Work out the finished part from the listing and answer in its coordinate system (mm). A direction names the side the tool comes from. Round coordinates to 2 decimals unless told otherwise and drop trailing zeros. Loops run counter-clockwise (first coordinate to the right, second up) from the corner with the lowest first, then second, coordinate; pieces in that order, holes last. Notation, with made-up numbers: (17, 3) - (44, 3) arc R30 cw to (44, 25) - close; hole circle Ø7 at (-27, 57.5). An arc over 180 degrees is marked (long way). Return JSON: item names as keys, results as strings.
from build123d import *

# Parameters (mm, degrees)
SKETCH1_W             = 50
SKETCH1_H             = 50
BOSS_EXTRUDE1_DEPTH   = 1810
BOSS_EXTRUDE1_2_DEPTH = 1810
BOSS_EXTRUDE1_3_DEPTH = 1810
BOSS_EXTRUDE1_4_DEPTH = 1810
BOSS_EXTRUDE2_START   = 10
SKETCH2_W             = 50
SKETCH2_H             = 750
SKETCH2_W_2           = 750
SKETCH2_H_2           = 100
BOSS_EXTRUDE2_DEPTH   = 180
SKETCH4_W             = 750
SKETCH4_H             = 110
CUT_EXTRUDE4_DEPTH    = 1050
SKETCH5_W             = 50
SKETCH5_H             = 50
SKETCH5_H_2           = 60
BOSS_EXTRUDE3_DEPTH   = 770
SKETCH6_W             = 50
SKETCH6_H             = 60
BOSS_EXTRUDE4_DEPTH   = 770
SKETCH8_W             = 50
SKETCH8_H             = 50
BOSS_EXTRUDE5_DEPTH   = 770
SKETCH9_W             = 50
SKETCH9_H             = 30
BOSS_EXTRUDE6_DEPTH   = 770
SKETCH10_R            = 15
BOSS_EXTRUDE7_DEPTH   = 770
SKETCH11_W            = 50
SKETCH11_H            = 30
BOSS_EXTRUDE8_DEPTH   = 770
SKETCH12_W            = 50
SKETCH12_H            = 30
BOSS_EXTRUDE9_DEPTH   = 770


with BuildPart() as part:
    # Sketch1 → Boss-Extrude1 (new body)
    with BuildSketch(Plane(origin=(0, 0, 0), x_dir=(1, 0, 0), z_dir=(0, 1, 0))):
        with Locations((-427.760736196, -623.312883436)):
            Rectangle(SKETCH1_W, SKETCH1_H)
    extrude(amount=BOSS_EXTRUDE1_DEPTH)



with BuildPart() as body_2:
    # Sketch1 → Boss-Extrude1 2 (new body)
    with BuildSketch(Plane(origin=(0, 0, 0), x_dir=(1, 0, 0), z_dir=(0, 1, 0))):
        with Locations((372.239263804, -623.312883436)):
            Rectangle(SKETCH1_W, SKETCH1_H)
    extrude(amount=BOSS_EXTRUDE1_2_DEPTH)


with BuildPart() as body_3:
    # Sketch1 → Boss-Extrude1 3 (new body)
    with BuildSketch(Plane(origin=(0, 0, 0), x_dir=(1, 0, 0), z_dir=(0, 1, 0))):
        with Locations((372.239263804, 176.687116564)):
            Rectangle(SKETCH1_W, SKETCH1_H)
    extrude(amount=BOSS_EXTRUDE1_3_DEPTH)


with BuildPart() as body_4:
    # Sketch1 → Boss-Extrude1 4 (new body)
    with BuildSketch(Plane(origin=(0, 0, 0), x_dir=(1, 0, 0), z_dir=(0, 1, 0))):
        with Locations((-427.760736196, 176.687116564)):
            Rectangle(SKETCH1_W, SKETCH1_H)
    extrude(amount=BOSS_EXTRUDE1_4_DEPTH)


with BuildPart() as part_1:
    add(part.part)

    add(body_2.part)  # Boss-Extrude2 merges body 2

    add(body_3.part)  # Boss-Extrude2 merges body 3

    add(body_4.part)  # Boss-Extrude2 merges body 4
    # Sketch2 → Boss-Extrude2 (add)
    with BuildSketch(Plane(origin=(0, 0, 0), x_dir=(-1, 0, 0), z_dir=(0, -1, 0)).offset(BOSS_EXTRUDE2_START)):
        with Locations((427.760736196, -223.312883436)):
            Rectangle(SKETCH2_W, SKETCH2_H)
        with Locations((27.760736196, -223.312883436)):
            Rectangle(SKETCH2_W_2, SKETCH2_H_2)
        with Locations((-372.239263804, -223.312883436)):
            Rectangle(SKETCH2_W, SKETCH2_H)
    extrude(amount=-BOSS_EXTRUDE2_DEPTH)

    # Sketch4 → Cut-Extrude4 (cut)
    with BuildSketch(Plane.ZY.offset(452.760736196)):
        with Locations((223.312883436, 45)):
            Rectangle(SKETCH4_W, SKETCH4_H)
    extrude(amount=-CUT_EXTRUDE4_DEPTH, mode=Mode.SUBTRACT)

    # Sketch5 → Boss-Extrude3 (add)
    with BuildSketch(Plane.ZY.offset(-347.239263804)):
        with Locations((-176.687116564, 940)):
            Rectangle(SKETCH5_W, SKETCH5_H)
        with Locations((623.312883436, 935)):
            Rectangle(SKETCH5_W, SKETCH5_H_2)
    extrude(amount=BOSS_EXTRUDE3_DEPTH)

    # Sketch6 → Boss-Extrude4 (add)
    with BuildSketch(Plane(origin=(0, 0, 598.312883436), x_dir=(-1, 0, 0), z_dir=(0, 0, -1))):
        with Locations((-372.239263804, 935)):
            Rectangle(SKETCH6_W, SKETCH6_H)
        with Locations((427.760736196, 935)):
            Rectangle(SKETCH6_W, SKETCH6_H)
    extrude(amount=BOSS_EXTRUDE4_DEPTH)

    # Sketch8 → Boss-Extrude5 (add)
    with BuildSketch(Plane(origin=(0, 0, 598.312883436), x_dir=(-1, 0, 0), z_dir=(0, 0, -1))):
        with Locations((-372.239263804, 1514.740067664)):
            Rectangle(SKETCH8_W, SKETCH8_H)
        with Locations((427.760736196, 1514.740067664)):
            Rectangle(SKETCH8_W, SKETCH8_H)
    extrude(amount=BOSS_EXTRUDE5_DEPTH)

    # Sketch9 → Boss-Extrude6 (add)
    with BuildSketch(Plane.XY.offset(-151.687116564)):
        with Locations((-427.760736196, 1795)):
            Rectangle(SKETCH9_W, SKETCH9_H)
        with Locations((372.239263804, 1795)):
            Rectangle(SKETCH9_W, SKETCH9_H)
    extrude(amount=BOSS_EXTRUDE6_DEPTH)

    # Sketch10 → Boss-Extrude7 (add)
    with BuildSketch(Plane(origin=(-402.760736196, 0, 0), x_dir=(0, 0, -1), z_dir=(1, 0, 0))):
        with Locations(Location((-223.312883436, 1795, 0), (0, 0, 270))):
            Circle(SKETCH10_R)
    extrude(amount=BOSS_EXTRUDE7_DEPTH)

    # Sketch11 → Boss-Extrude8 (add)
    with BuildSketch(Plane.ZY.offset(-347.239263804)):
        with Locations((-176.687116564, 1795)):
            Rectangle(SKETCH11_W, SKETCH11_H)
    extrude(amount=BOSS_EXTRUDE8_DEPTH)

    # Sketch12 → Boss-Extrude9 (add)
    with BuildSketch(Plane.ZY.offset(-347.239263804)):
        with Locations((-176.687116564, 384.816862376)):
            Rectangle(SKETCH12_W, SKETCH12_H)
    extrude(amount=BOSS_EXTRUDE9_DEPTH)


solid = part_1.part
1) A flat-ended cylindrical pin translates along its axis: pin 1 (15 mm diameter, centred on x = -421.5, z = 200.5, fed in from -Y). Find the tip coordinate at first contact, or state that the pin passes through.
Verdict:
{"pin 1": "stops at y = 100"}
2) Section A-A (y = 1509) is taken. Give the vertices of the cut face in (x, z).
Verdict:
{"outline": "(-452.76, -201.69) - (-402.76, -201.69) - (-402.76, 648.31) - (-452.76, 648.31) - close; (347.24, -201.69) - (397.24, -201.69) - (397.24, 648.31) - (347.24, 648.31) - close"}
3) Find the intervals of material crossed by L1, parallel to X at y = 916.5, z = 541; L2, parallel to Y at x = -337, z = 261; L3, parallel to Z at x = -52.5, y = 148.5, in increasing order.
Verdict:
{"L1": "x = -452.76 to -402.76, 347.24 to 397.24", "L2": "y = 100 to 170", "L3": "z = 173.31 to 273.31"}
4) Section D-D (x = -357.5) is taken. Give the vertices of the cut face in (y, z).
Verdict:
{"outline": "(100, 173.31) - (170, 173.31) - (170, 273.31) - (100, 273.31) - close; (369.82, -201.69) - (399.82, -201.69) - (399.82, -151.69) - (369.82, -151.69) - close; (905, 598.31) - (965, 598.31) - (965, 648.31) - (905, 648.31) - close; (915, -201.69) - (965, -201.69) - (965, -151.69) - (915, -151.69) - close; (1780, -201.69) - (1810, -201.69) - (1810, -151.69) - (1780, -151.69) - close; circle Ø30 at (1795, 223.31)"}
5) A tool of negligible diameter and unlimited length cuts with its end or side. For faces 1 (the flat face through (372, 1780, 218)), 2 (the flat face through (-23, 965, 623)), 3 (the flat face through (-33, 935, 598.313)), 4 (the flat face through (-23, 135, 273.313)), from which of +Z, -Z, +X, -X, +Y, -Y can it reach the whole face along a straight path? Write none if from no direction.
Verdict:
{"face 1": "+X, -X", "face 2": "+Z, -Z, +Y", "face 3": "+Y, -Y", "face 4": "+Z, +Y, -Y"}
6) Section C-C (y = 1244.5) is taken. Give the vertices of the cut face in (x, z), and give its area (3 significant figures).
Verdict:
{"outline": "(-452.76, -201.69) - (-402.76, -201.69) - (-402.76, -151.69) - (-452.76, -151.69) - close; (-452.76, 598.31) - (-402.76, 598.31) - (-402.76, 648.31) - (-452.76, 648.31) - close; (347.24, -201.69) - (397.24, -201.69) - (397.24, -151.69) - (347.24, -151.69) - close; (347.24, 598.31) - (397.24, 598.31) - (397.24, 648.31) - (347.24, 648.31) - close", "area": "10,000 mm2"}
7) Section B-B (z = 118) is taken. Count the separate pieces of the cut face and the enclosed holes in it, and give its area (3 significant figures).
Verdict:
{"separate pieces": "8", "enclosed holes": "0", "area": "21,000 mm2"}
8) Determine the mould class of faces 5 (the flat face through (372, 1224, 598.313)), 6 (the flat face through (-452.761, 834, 599)), 7 (the flat face through (-23, 135, 173.313)) for opening direction Z: pulls with the +Z half, pulls with the -Z half, needs draft (parallel to the pull), parting line crosses it, or undercut.
Verdict:
{"face 5": "undercut", "face 6": "needs draft", "face 7": "pulls with the -Z half"}
